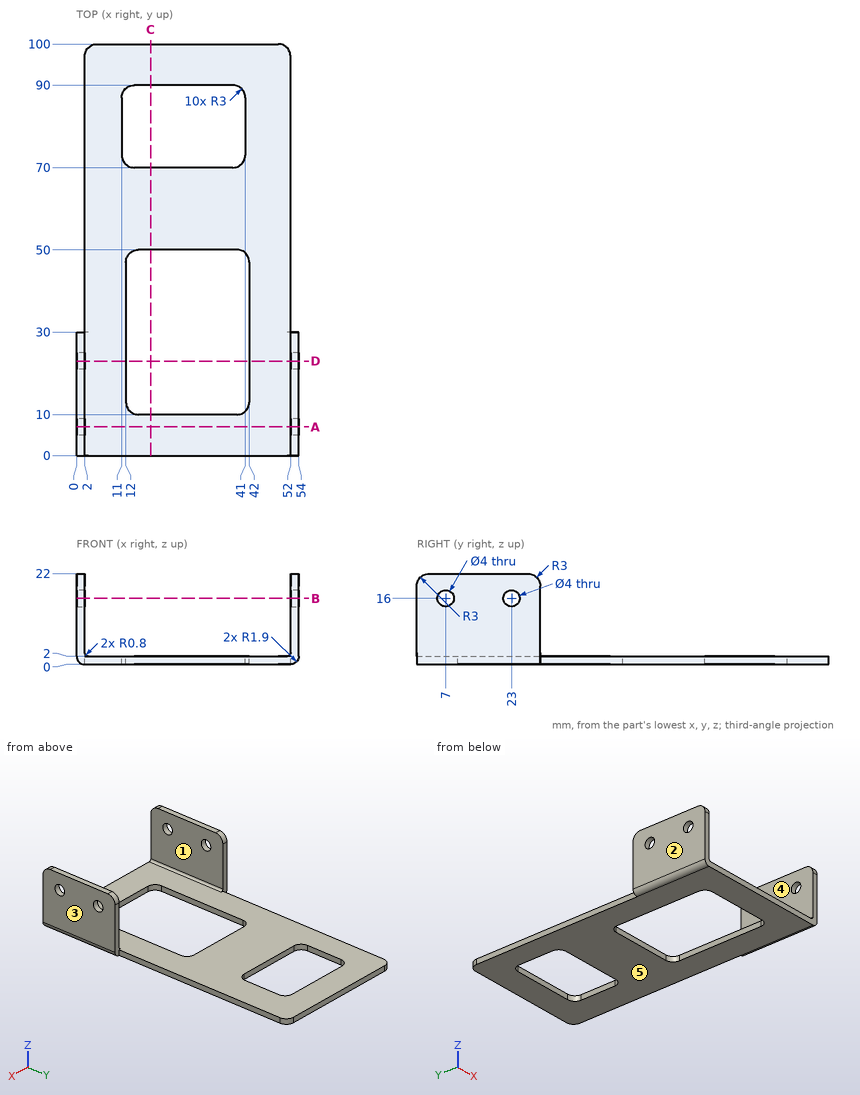
Design review of the part shown in the three views and the two pictorial views. Dimensions are in mm from the part's minimum x, y and z. A direction names the side the tool comes from. Give positions to 0.01 mm unless a question says otherwise; leave off trailing zeros. Loops run counter-clockwise (first coordinate to the right, second up) from the corner with the lowest first, then second, coordinate; pieces in that order, holes last. Notation, with made-up numbers: (84, 25) -> (142, 25) arc R23 ccw to (142, 59) -> close; hole circle Ø7 at (52.25, 72). An arc over 180 degrees is marked (long way). Write each question's results on one line, items separated by ' | '.
Q1. Take a section at A-A, the plane y = 7. Write out the cut boundary in (x, z), plus the area to 3 significant figures.
Reply:
outline: (0, 1.9) arc R1.9 ccw to (1.9, 0) -> (52.1, 0) arc R1.9 ccw to (54, 1.9) -> (54, 14) -> (52, 14) -> (52, 2.8) arc R0.8 cw to (51.2, 2) -> (2.8, 2) arc R0.8 cw to (2, 2.8) -> (2, 14) -> (0, 14) -> close; (0, 18) -> (2, 18) -> (2, 22) -> (0, 22) -> close; (52, 18) -> (54, 18) -> (54, 22) -> (52, 22) -> close | area: 171 mm²
Q2. Take a section at C-C, the plane x = 18. Write out the cut boundary in (y, z), plus the area to 3 significant figures.
Reply:
outline: (0, 0) -> (10, 0) -> (10, 2) -> (0, 2) -> close; (50, 0) -> (70, 0) -> (70, 2) -> (50, 2) -> close; (90, 0) -> (100, 0) -> (100, 2) -> (90, 2) -> close | area: 80.0 mm²
Q3. The part is to be moulded in two halves that separate along X. For the marked faces 3, 4 and 5, say which applies: +X half, -X half, draft (parallel to the pull), parting line (faces both ways), or undercut.
Reply:
face 3: +X half | face 4: undercut | face 5: draft
Q4. Machinability: for the marked faces 1 and 2, which of the approach directions +Z, -Z, +X, -X, +Y, -Y give a long, thin tool a straight path to every point of the face, cutting with its end or side? Answer none if there is none.
Reply:
face 1: +Z, +Y, -Y | face 2: +Z, -Z, -X, +Y, -Y
Q5. Take a section at B-B, the plane z = 16. Write out the cut boundary in (x, y), plus the area to 3 significant figures.
Reply:
outline: (0, 0) -> (2, 0) -> (2, 5) -> (0, 5) -> close; (0, 9) -> (2, 9) -> (2, 21) -> (0, 21) -> close; (0, 25) -> (2, 25) -> (2, 30) -> (0, 30) -> close; (52, 0) -> (54, 0) -> (54, 5) -> (52, 5) -> close; (52, 9) -> (54, 9) -> (54, 21) -> (52, 21) -> close; (52, 25) -> (54, 25) -> (54, 30) -> (52, 30) -> close | area: 88.0 mm²
Q6. For pin 1 Ø25 at (x, y) = (24, 37.5) entering from +Z; pin 2 Ø10 at (x, y) = (17, 77) entering from +Z; pin 3 Ø0.6 at (y, z) = (78, 1) entering from -X; pin 4 Ø0.6 at (y, z) = (82.5, 0.5) entering from +X, all flat-tipped, find the tip position at first contact; note any pin that passes through.
Reply:
pin 1: stops at z = 2 | pin 2: passes through | pin 3: stops at x = 2 | pin 4: stops at x = 52
Q7. Take a section at D-D, the plane y = 23. Write out the cut boundary in (x, z).
Reply:
outline: (0, 1.9) arc R1.9 ccw to (1.9, 0) -> (12, 0) -> (12, 2) -> (2.8, 2) arc R0.8 cw to (2, 2.8) -> (2, 14) -> (0, 14) -> close; (0, 18) -> (2, 18) -> (2, 22) -> (0, 22) -> close; (42, 0) -> (52.1, 0) arc R1.9 ccw to (54, 1.9) -> (54, 14) -> (52, 14) -> (52, 2.8) arc R0.8 cw to (51.2, 2) -> (42, 2) -> close; (52, 18) -> (54, 18) -> (54, 22) -> (52, 22) -> close
Q8. Wall thickness on L1, parallel to Y at x = 1.5, z = 16; L2, parallel to X at y = 29.5, z = 9; L3, parallel to Z at x = 0.6, y = 23: over which ranges is each line inside the solid? List them lowest first.
Reply:
L1: y = 0 to 5, 9 to 21, 25 to 30 | L2: x = 0 to 2, 52 to 54 | L3: z = 0.51 to 14, 18 to 22
